```python
from build123d import *

# Parameters (mm, degrees)
BOSS_EXTRUDE1_DEPTH = 1828.8
THRU_HOLES_D        = 3.4544


with BuildPart() as part:
    # Sketch1 → Boss-Extrude1 (new body)
    with BuildSketch(Plane(origin=(0, 0, 0), x_dir=(1, 0, 0), z_dir=(0, 1, 0))):
        with BuildLine():
            Line((-4.445, 17.018), (-4.445, 4.953))
            ThreePointArc((-4.445, 4.953), (-4.482197439, 4.863197439), (-4.572, 4.826))
            Line((-4.572, 4.826), (-7.366, 4.826))
            ThreePointArc((-7.366, 4.826), (-7.545605122, 4.751605122), (-7.62, 4.572))
            Line((-7.62, 4.572), (-7.62, 0))
            ThreePointArc((-7.62, 0), (-5.388153673, -5.388153673), (0, -7.62))
            Line((0, -7.62), (4.572, -7.62))
            ThreePointArc((4.572, -7.62), (4.751605122, -7.545605122), (4.826, -7.366))
            Line((4.826, -7.366), (4.826, -4.572))
            ThreePointArc((4.826, -4.572), (4.863197439, -4.482197439), (4.953, -4.445))
            Line((4.953, -4.445), (17.018, -4.445))
            ThreePointArc((17.018, -4.445), (17.556815367, -4.221815367), (17.78, -3.683))
            Line((17.78, -3.683), (17.78, 1.143))
            ThreePointArc((17.78, 1.143), (17.556815367, 1.681815367), (17.018, 1.905))
            Line((17.018, 1.905), (4.87752755, 1.905))
            ThreePointArc((4.87752755, 1.905), (4.73895919, 1.946127246), (4.645264333, 2.056190476))
            ThreePointArc((4.645264333, 2.056190476), (3.592102448, 3.592102448), (2.056190476, 4.645264333))
            ThreePointArc((2.056190476, 4.645264333), (1.946127246, 4.73895919), (1.905, 4.87752755))
            Line((1.905, 4.87752755), (1.905, 17.018))
            ThreePointArc((1.905, 17.018), (1.681815367, 17.556815367), (1.143, 17.78))
            Line((1.143, 17.78), (-3.683, 17.78))
            ThreePointArc((-3.683, 17.78), (-4.221815367, 17.556815367), (-4.445, 17.018))
        make_face()
    extrude(amount=BOSS_EXTRUDE1_DEPTH)

    # THRU HOLES (through all)
    with Locations(Plane(origin=(0, 1828.8, 0), x_dir=(1, 0, 0), z_dir=(0, 1, 0))):
        with Locations((0, 0)):
            Hole(THRU_HOLES_D / 2)


solid = part.part
```
Model file for the job. Use its own axes, mm. Coordinates: 2 decimals unless noted, no trailing zeros. Write each loop counter-clockwise with the first axis right and the second up, starting at its lowest first coordinate (ties: lowest second). Pieces come first, ordered by that corner, then holes. Notation, with made-up numbers: (54.25, -12.75) - (109.25, -12.75) arc R13 ccw to (109.25, 0.25) - close; hole circle Ø2 at (4.25, -4.5). An arc over 180 degrees is marked (long way). Use a Markdown table: item, result. Add a question column.
Item 1: Band-saw the part on A-A, the plane y = 1265. Write the cut outline in (x, z) (3 decimals), and give its area (3 significant figures).
Item 2: Drop flat-ended pins along their axis: pin 1 (5 mm diameter, centred on x = 8, y = 1389, fed in from +Z) (3 decimals); pin 2 (6 mm diameter, centred on x = 11.5, y = 478.5, fed in from -Z) (3 decimals); pin 3 (9.5 mm diameter, centred on x = 8.5, y = 700.5, fed in from +Z); pin 4 (3.5 mm diameter, centred on y = 506.5, z = -11.5, fed in from +X) (3 decimals). Give the stop position or say it passes through.
Item 3: Band-saw the part on B-B, the plane x = 13. Write the cut outline in (y, z) (3 decimals), and give its area (3 significant figures).
Item 4: Drill centre lines: line 1 along Z through (x, y) = (0, 984); line 2 along Z through (x, y) = (1.5, 1668.5); line 3 along X through (y, z) = (1417.5, -12.75) (3 decimals). Where is each one in solid material? Low to high.
A:
| question | item | result |
|---|---|---|
| 1 | outline | (-7.62, -4.572) arc R0.254 ccw to (-7.366, -4.826) - (-4.572, -4.826) arc R0.127 cw to (-4.445, -4.953) - (-4.445, -17.018) arc R0.762 ccw to (-3.683, -17.78) - (1.143, -17.78) arc R0.762 ccw to (1.905, -17.018) - (1.905, -4.878) arc R0.254 cw to (2.056, -4.645) arc R5.08 ccw to (4.645, -2.056) arc R0.254 cw to (4.878, -1.905) - (17.018, -1.905) arc R0.762 ccw to (17.78, -1.143) - (17.78, 3.683) arc R0.762 ccw to (17.018, 4.445) - (4.953, 4.445) arc R0.127 cw to (4.826, 4.572) - (4.826, 7.366) arc R0.254 ccw to (4.572, 7.62) - (0, 7.62) arc R7.62 ccw to (-7.62, 0) - close; hole circle Ø3.454 at (0, 0) |
| 1 | area | 294 mm² |
| 2 | pin 1 | stops at z = 4.445 |
| 2 | pin 2 | stops at z = -1.905 |
| 2 | pin 3 | stops at z = 7.62 |
| 2 | pin 4 | stops at x = 1.905 |
| 3 | outline | (0, -1.905) - (1828.8, -1.905) - (1828.8, 4.445) - (0, 4.445) - close |
| 3 | area | 11,600 mm² |
| 4 | line 1 | z = -17.78 to -1.73, 1.73 to 7.62 |
| 4 | line 2 | z = -17.69 to -0.86, 0.86 to 7.62 |
| 4 | line 3 | x = -4.445 to 1.905 |
